from build123d import *

# Parameters (mm, degrees)
SKETCH2_R                        = 139.7
SKETCH2_R_2                      = 31.75
BOSS_EXTRUDE1_DEPTH              = 9.525
SKETCH3_R                        = 3.175
SKETCH3_R_2                      = 6.35
CUT_EXTRUDE2_DEPTH               = 10.525
F_1_2_20_TAPPED_HOLE1_AT_2_COUNT = 2
F_1_2_20_TAPPED_HOLE1_AT_2_PITCH = 170.6248663
F_1_2_20_TAPPED_HOLE1_AT_3_COUNT = 2
F_1_2_20_TAPPED_HOLE1_AT_3_PITCH = 241.3
F_1_2_20_TAPPED_HOLE1_AT_4_COUNT = 2
F_1_2_20_TAPPED_HOLE1_AT_4_PITCH = 170.6248663


with BuildPart() as part:
    # Sketch2 → Boss-Extrude1 (new body)
    with BuildSketch(Plane(origin=(0, 0, 0), x_dir=(1, 0, 0), z_dir=(0, 1, 0))):
        Circle(SKETCH2_R)
        Circle(SKETCH2_R_2, mode=Mode.SUBTRACT)
        with BuildLine():
            Line((61.954602754, 26.03357827), (81.460512242, 45.539487758))
            ThreePointArc((81.460512242, 45.539487758), (87.024437868, 47.307910551), (91.68068299, 43.785983677))
            ThreePointArc((91.68068299, 43.785983677), (101.6, 0), (91.68068299, -43.785983677))
            ThreePointArc((91.68068299, -43.785983677), (87.024437868, -47.307910551), (81.460512242, -45.539487758))
            Line((81.460512242, -45.539487758), (61.954602754, -26.03357827))
            ThreePointArc((61.954602754, -26.03357827), (60.270643836, -23.027751383), (60.404300741, -19.584954736))
            ThreePointArc((60.404300741, -19.584954736), (63.5, 0), (60.404300741, 19.584954736))
            ThreePointArc((60.404300741, 19.584954736), (60.270643836, 23.027751383), (61.954602754, 26.03357827))
        make_face(mode=Mode.SUBTRACT)
        with BuildLine():
            Line((26.03357827, 61.954602754), (45.539487758, 81.460512242))
            ThreePointArc((45.539487758, 81.460512242), (47.307910551, 87.024437868), (43.785983677, 91.68068299))
            ThreePointArc((43.785983677, 91.68068299), (0, 101.6), (-43.785983677, 91.68068299))
            ThreePointArc((-43.785983677, 91.68068299), (-47.307910551, 87.024437868), (-45.539487758, 81.460512242))
            Line((-45.539487758, 81.460512242), (-26.03357827, 61.954602754))
            ThreePointArc((-26.03357827, 61.954602754), (-23.027751383, 60.270643836), (-19.584954736, 60.404300741))
            ThreePointArc((-19.584954736, 60.404300741), (0, 63.5), (19.584954736, 60.404300741))
            ThreePointArc((19.584954736, 60.404300741), (23.027751383, 60.270643836), (26.03357827, 61.954602754))
        make_face(mode=Mode.SUBTRACT)
        with BuildLine():
            Line((26.03357827, -61.954602754), (45.539487758, -81.460512242))
            ThreePointArc((45.539487758, -81.460512242), (47.307910551, -87.024437868), (43.785983677, -91.68068299))
            ThreePointArc((43.785983677, -91.68068299), (0, -101.6), (-43.785983677, -91.68068299))
            ThreePointArc((-43.785983677, -91.68068299), (-47.307910551, -87.024437868), (-45.539487758, -81.460512242))
            Line((-45.539487758, -81.460512242), (-26.03357827, -61.954602754))
            ThreePointArc((-26.03357827, -61.954602754), (-23.027751383, -60.270643836), (-19.584954736, -60.404300741))
            ThreePointArc((-19.584954736, -60.404300741), (0, -63.5), (19.584954736, -60.404300741))
            ThreePointArc((19.584954736, -60.404300741), (23.027751383, -60.270643836), (26.03357827, -61.954602754))
        make_face(mode=Mode.SUBTRACT)
        with BuildLine():
            Line((-61.954602754, -26.03357827), (-81.460512242, -45.539487758))
            ThreePointArc((-81.460512242, -45.539487758), (-87.024437868, -47.307910551), (-91.68068299, -43.785983677))
            ThreePointArc((-91.68068299, -43.785983677), (-101.6, 0), (-91.68068299, 43.785983677))
            ThreePointArc((-91.68068299, 43.785983677), (-87.024437868, 47.307910551), (-81.460512242, 45.539487758))
            Line((-81.460512242, 45.539487758), (-61.954602754, 26.03357827))
            ThreePointArc((-61.954602754, 26.03357827), (-60.270643836, 23.027751383), (-60.404300741, 19.584954736))
            ThreePointArc((-60.404300741, 19.584954736), (-63.5, 0), (-60.404300741, -19.584954736))
            ThreePointArc((-60.404300741, -19.584954736), (-60.270643836, -23.027751383), (-61.954602754, -26.03357827))
        make_face(mode=Mode.SUBTRACT)
    extrude(amount=BOSS_EXTRUDE1_DEPTH)

    # Sketch3 → Cut-Extrude2 (cut, through all)
    with BuildSketch(Plane(origin=(0, 9.525, 0), x_dir=(1, 0, 0), z_dir=(0, 1, 0))):
        with Locations((-71.842048969, 71.842048969)):
            Circle(SKETCH3_R)
        with Locations((-53.881536726, 53.881536726)):
            Circle(SKETCH3_R)
        with Locations((-71.842048969, -71.842048969)):
            Circle(SKETCH3_R)
        with Locations((71.842048969, -71.842048969)):
            Circle(SKETCH3_R)
        with Locations((71.842048969, 71.842048969)):
            Circle(SKETCH3_R)
        with Locations((53.881536726, 53.881536726)):
            Circle(SKETCH3_R)
        with Locations((53.881536726, -53.881536726)):
            Circle(SKETCH3_R)
        with Locations((-53.881536726, -53.881536726)):
            Circle(SKETCH3_R)
        with Locations((85.31243315, 85.31243315)):
            Circle(SKETCH3_R_2)
        with Locations((85.31243315, -85.31243315)):
            Circle(SKETCH3_R_2)
        with Locations((-85.31243315, -85.31243315)):
            Circle(SKETCH3_R_2)
        with Locations((-85.31243315, 85.31243315)):
            Circle(SKETCH3_R_2)
    extrude(amount=-CUT_EXTRUDE2_DEPTH, mode=Mode.SUBTRACT)

    # Sketch7 → 1/2-20 Tapped Hole1 (revolve, cut)
    with BuildSketch(Plane(origin=(-120.65, 9.525, 0), x_dir=(0, 0, 1), z_dir=(1, 0, 0))):
        Polygon((0, 0), (0, 9.525), (6.985, 9.525), (5.75437, 8.29437), (5.75437, 1.23063), (6.985, 0), align=None)
    f_1_2_20_tapped_hole1 = revolve(axis=Axis((-120.65, 15.875, 0), (0, -1, 0)), mode=Mode.SUBTRACT)

    # 1/2-20 Tapped Hole1 at 2: 1/2-20 Tapped Hole1 ×2
    with Locations(*[Vector(0.707106781, 0, -0.707106781) * (i * F_1_2_20_TAPPED_HOLE1_AT_2_PITCH) for i in range(1, F_1_2_20_TAPPED_HOLE1_AT_2_COUNT)]):
        add(f_1_2_20_tapped_hole1, mode=Mode.SUBTRACT)

    # 1/2-20 Tapped Hole1 at 3: 1/2-20 Tapped Hole1 ×2
    with Locations(*[(i * F_1_2_20_TAPPED_HOLE1_AT_3_PITCH, 0, 0) for i in range(1, F_1_2_20_TAPPED_HOLE1_AT_3_COUNT)]):
        add(f_1_2_20_tapped_hole1, mode=Mode.SUBTRACT)

    # 1/2-20 Tapped Hole1 at 4: 1/2-20 Tapped Hole1 ×2
    with Locations(*[Vector(0.707106781, 0, 0.707106781) * (i * F_1_2_20_TAPPED_HOLE1_AT_4_PITCH) for i in range(1, F_1_2_20_TAPPED_HOLE1_AT_4_COUNT)]):
        add(f_1_2_20_tapped_hole1, mode=Mode.SUBTRACT)


solid = part.part
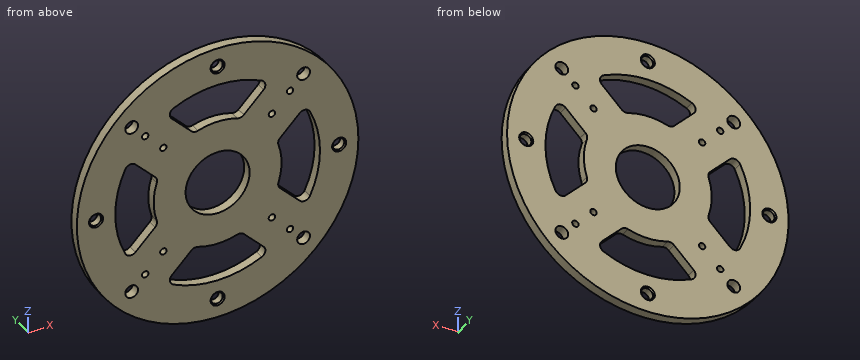
Can you work these out from the model? Positions are in its coordinate system, mm. Round coordinates to 2 decimals unless told otherwise and drop trailing zeros. Loops run counter-clockwise (first coordinate to the right, second up) from the corner with the lowest first, then second, coordinate; pieces in that order, holes last. Notation, with made-up numbers: (-8.5, 2) - (36.5, 2) arc R35 ccw to (36.5, 38) - close; hole circle Ø11 at (82, -24.75). An arc over 180 degrees is marked (long way). Write item = value, one per line. Start each with the question number.
(1) If I drill on probe 1 along Z at (x, y) = (0, 6.5); probe 2 along Z at (x, y) = (-71, 7); probe 3 along X at (y, z) = (2.75, 43.5), over which ranges is the centre line in solid material (lowest first)? Write a range as [from, to].
(2) If we section it at D-D (z = 96.5): Please give me the cut outline in (x, y) (3 decimals), and give its area (3 significant figures).
(3) For P1, Ø6, axis at x = -95.5, z = -64, coming from the -Y side; P2, Ø13, axis at x = 120.65, z = 0, coming from the -Y side (3 decimals); P3, Ø5, axis at y = 1.5, z = 56.5, coming from the +X side; P4, Ø3, axis at x = -8, y = 4, coming from the -Z side, each with a flat end and sliding along its axis, tell me the tip position at first contact or that it passes through.
(4) If we section it at A-A (x = 0): Give the number of separate pieces and of enclosed holes in the cut face, and give its area (3 significant figures).
(5) If we section it at C-C (x = -120.65): Please give me the cut outline in (y, z) (3 decimals), and give its area (3 significant figures).
Ans:
q1.probe_1 = [-139.7, -126.4], [-114.9, -101.6], [-63.5, -31.75], [31.75, 63.5], [101.6, 114.9], [126.4, 139.7]
q1.probe_2 = [-120.31, -74.9], [-68.78, -35.08], [35.08, 68.78], [74.9, 120.31]
q1.probe_3 = [-132.75, -91.82], [-79.42, 79.42], [91.82, 132.75]
q2.outline = (-101.014, 0) - (-31.785, 0) - (-31.785, 9.525) - (-101.014, 9.525) - close; (31.785, 0) - (101.014, 0) - (101.014, 9.525) - (31.785, 9.525) - close
q2.area = 1,320 mm²
q3.P1 = 0
q3.P2 = 0.485
q3.P3 = 128.84
q3.P4 = -139.55
q4.separate_pieces = 6
q4.enclosed_holes = 0
q4.area = 1,110 mm²
q5.outline = (0, -70.425) - (9.525, -70.425) - (9.525, -6.985) - (8.294, -5.754) - (1.231, -5.754) - (0, -6.985) - close; (0, 6.985) - (1.231, 5.754) - (8.294, 5.754) - (9.525, 6.985) - (9.525, 70.425) - (0, 70.425) - close
q5.area = 1,230 mm²
